For this review, use the dimensioned drawing (mm, ordinates from the lowest corner) and the shaded views. Round coordinates to 2 decimals unless told otherwise and drop trailing zeros. Order: outer loops, then holes, each group sorted by start corner. A loop starts at its lowest first (then second) coordinate and runs counter-clockwise, first axis right, second up. Notation, with made-up numbers: M -32.75,29.25 L -19.75,29.25 A22 ccw -19.75,47.25 Z; hole C 71,85.25 d8. An arc over 180 degrees is marked long. Use a Markdown table: item, result. Add a question column.
1. Consider section A-A on x = 36. State the section outline as (y, z) points, then the cut area to 3 significant figures.
2. Consider section D-D on z = 7.5. State the section outline as (x, y) points, then the cut area to 3 significant figures.
3. To check wall thickness, follow probe 1 along Z at (x, y) = (36, 2.3); probe 2 along X at (y, z) = (0.7, 15.5); probe 3 along Z at (x, y) = (14.5, 1.45). State the ranges of each line that lie inside material, in increasing order.
4. Consider section C-C on y = 1.35. State the section outline as (x, z) points, then the cut area to 3 significant figures.
5. Consider section B-B on z = 3. State the section outline as (x, y) points, then the cut area to 3 significant figures.
6. Insertion check: P1, Ø2.5, axis at x = 15, z = 15.5, coming from the -Y side; P2, Ø1, axis at y = 1.5, z = 7, coming from the +X side. Each pin has a flat end and moves straight along its axis. Give the tip position at first contact, or say it passes through.
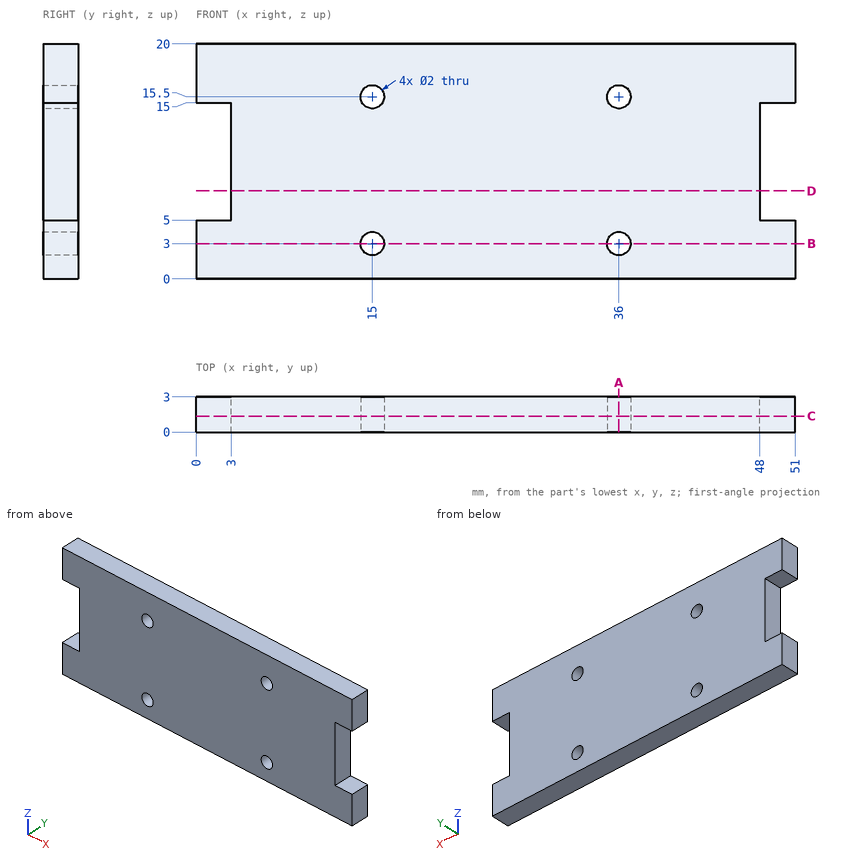
Answer block:
| question | item | result |
|---|---|---|
| 1 | outline | M 0,0 L 3,0 L 3,2 L 0,2 Z; M 0,4 L 3,4 L 3,14.5 L 0,14.5 Z; M 0,16.5 L 3,16.5 L 3,20 L 0,20 Z |
| 1 | area | 48.0 mm^2 |
| 2 | outline | M 3,0 L 48,0 L 48,3 L 3,3 Z |
| 2 | area | 135 mm^2 |
| 3 | probe 1 | 0 to 2, 4 to 14.5, 16.5 to 20 |
| 3 | probe 2 | 0 to 14, 16 to 35, 37 to 51 |
| 3 | probe 3 | 0 to 2.13, 3.87 to 14.63, 16.37 to 20 |
| 4 | outline | M 0,0 L 51,0 L 51,5 L 48,5 L 48,15 L 51,15 L 51,20 L 0,20 L 0,15 L 3,15 L 3,5 L 0,5 Z; hole C 15,3 d2; hole C 15,15.5 d2; hole C 36,3 d2; hole C 36,15.5 d2 |
| 4 | area | 947 mm^2 |
| 5 | outline | M 0,0 L 14,0 L 14,3 L 0,3 Z; M 16,0 L 35,0 L 35,3 L 16,3 Z; M 37,0 L 51,0 L 51,3 L 37,3 Z |
| 5 | area | 141 mm^2 |
| 6 | P1 | y = 0 |
| 6 | P2 | x = 48 |
